from build123d import *

# Parameters (mm, degrees)
SKETCH2_W           = 50
SKETCH2_H           = 50
BOSS_EXTRUDE1_DEPTH = 50
SKETCH3_W           = 25
SKETCH3_H           = 25
CUT_EXTRUDE1_DEPTH  = 76
SKETCH4_W           = 25
SKETCH4_H           = 25
CUT_EXTRUDE2_DEPTH  = 62.23724357
SKETCH5_W           = 25
SKETCH5_H           = 25
CUT_EXTRUDE3_DEPTH  = 76


with BuildPart() as part:
    # Sketch2 → Boss-Extrude1 (new body)
    with BuildSketch(Plane.XY):
        Rectangle(SKETCH2_W, SKETCH2_H)
    extrude(amount=BOSS_EXTRUDE1_DEPTH)

    # Sketch3 → Cut-Extrude1 (cut, through all)
    with BuildSketch(Plane(origin=(0, 25, 0), x_dir=(1, 0, 0), z_dir=(0, 1, 0))):
        with Locations((0, -25)):
            Rectangle(SKETCH3_W, SKETCH3_H)
    extrude(amount=-CUT_EXTRUDE1_DEPTH, mode=Mode.SUBTRACT)

    # Sketch4 → Cut-Extrude2 (cut, through all)
    with BuildSketch(Plane.XY.offset(50)):
        Rectangle(SKETCH4_W, SKETCH4_H)
    extrude(amount=-CUT_EXTRUDE2_DEPTH, mode=Mode.SUBTRACT)

    # Sketch5 → Cut-Extrude3 (cut, through all)
    with BuildSketch(Plane(origin=(25, 0, 0), x_dir=(0, 0, -1), z_dir=(1, 0, 0))):
        with Locations((-25, 0)):
            Rectangle(SKETCH5_W, SKETCH5_H)
    extrude(amount=-CUT_EXTRUDE3_DEPTH, mode=Mode.SUBTRACT)


solid = part.part
Design review of the part built by this model. Coordinates are the model's own, in mm. A direction names the side the tool comes from. Round coordinates to 2 decimals unless told otherwise and drop trailing zeros. Loops run counter-clockwise (first coordinate to the right, second up) from the corner with the lowest first, then second, coordinate; pieces in that order, holes last. Notation, with made-up numbers: (65.5, -31.75) -> (83.5, -31.75) arc R26 ccw to (83.5, -7.75) -> close; hole circle Ø9 at (77.25, -25). An arc over 180 degrees is marked (long way). Use one line per item in the form item = value. Start each with the question number.
Q1. We need section A-A on y = 7. Give the boundary of the cut face in (x, z), then the cut area to 3 significant figures.
Q2. Wall thickness on line 1 along Y through (x, z) = (-18.5, 20.5); line 2 along Z through (x, y) = (-17, 2): over which ranges is each line inside the solid? List them lowest first. Write a range as [from, to].
Q3. We need section D-D on x = -17. Give the boundary of the cut face in (y, z).
Q4. We need section C-C on z = 4.5. Give the boundary of the cut face in (x, y).
Q5. Draft analysis for pull direction Z (two halves, no side actions). For faces 5 (the face through (19, 0, 12.5)), 6 (the face through (0, -25, 41)), state which applies: +Z half, -Z half, draft (parallel to the pull), parting line (faces both ways), or undercut.
Q6. Machinability: for faces 1 (the face through (12.5, 0, 44)), 2 (the face through (-19, -12.5, 25)), 3 (the face through (25, 0, 41)), 4 (the face through (12.5, -19, 25)), which of the approach directions +Z, -Z, +X, -X, +Y, -Y give a long, thin tool a straight path to every point of the face, cutting with its end or side? Answer none if there is none.
Calculated:
q1.outline = (-25, 0) -> (-12.5, 0) -> (-12.5, 12.5) -> (-25, 12.5) -> close; (-25, 37.5) -> (-12.5, 37.5) -> (-12.5, 50) -> (-25, 50) -> close; (12.5, 0) -> (25, 0) -> (25, 12.5) -> (12.5, 12.5) -> close; (12.5, 37.5) -> (25, 37.5) -> (25, 50) -> (12.5, 50) -> close
q1.area = 625 mm²
q2.line_1 = [-25, -12.5], [12.5, 25]
q2.line_2 = [0, 12.5], [37.5, 50]
q3.outline = (-25, 0) -> (25, 0) -> (25, 50) -> (-25, 50) -> close; hole (-12.5, 12.5) -> (12.5, 12.5) -> (12.5, 37.5) -> (-12.5, 37.5) -> close
q4.outline = (-25, -25) -> (25, -25) -> (25, 25) -> (-25, 25) -> close; hole (-12.5, -12.5) -> (12.5, -12.5) -> (12.5, 12.5) -> (-12.5, 12.5) -> close
q5.face_5 = undercut
q5.face_6 = draft
q6.face_1 = +Z, -Z
q6.face_2 = +X, -X
q6.face_3 = +Z, -Z, +X, +Y, -Y
q6.face_4 = +Y, -Y
